Source: CAD feature listing. Evaluate the final solid. Frame: model axes, mm. A direction names the side the tool comes from. Coordinates: 2 decimals unless noted, no trailing zeros. Order: outer loops, then holes, each group sorted by start corner. A loop starts at its lowest first (then second) coordinate and runs counter-clockwise, first axis right, second up. Notation, with made-up numbers: (1.25, 27) -> (13.25, 27) arc R3 ccw to (13.25, 32) -> close; hole circle Ø3 at (21.5, 0). An arc over 180 degrees is marked (long way). Write item = value, one per line. Start each with the question number.
Item 1: Ray query, line 1 along X through (y, z) = (-7.25, -259); line 2 along X through (y, z) = (-26.5, 47.5). Return the intervals inside material, ascending. Write a range as [from, to].
Item 2: Section query B-B (z = -304). Output: boundary loops of the cut face in (x, y), then the cut area to 3 significant figures.
Item 3: Set-up query: faces 1 (the flat face through (30, -15, -228)), 2 (the flat face through (15, -15, -450)). Return all of +Z, -Z, +X, -X, +Y, -Y with unobstructed straight access to the full face (end or side cutting, diameter ignored); none if empty.
Item 4: Contact query for flat-ended pins moving along their axis: pin 1 (4 mm diameter, centred on x = 67.5, z = 369.5, fed in from +Y); pin 2 (10 mm diameter, centred on y = -10, z = 57, fed in from +X); pin 3 (9 mm diameter, centred on y = -5, z = -35.5, fed in from +X). Output: stop coordinate, or through.
Item 5: Section query A-A (y = -14.75). Output: boundary loops of the cut face in (x, z).
Item 6: Section query C-C (z = 126). Output: boundary loops of the cut face in (x, y), then the cut area to 3 significant figures.
```python
from build123d import *

# Parameters (mm, degrees)
F1_DEPTH = 30
F3_DEPTH = 8
F4_W     = 10
F4_H     = 30
F5_DEPTH = 8
F6_W     = 10
F6_H     = 30
F7_DEPTH = 8


with BuildPart() as f1:
    # F0 (on Front) → F1 (new body)
    with BuildSketch(Plane.XZ):
        Polygon((70.294598, 500), (0, 0), (0, -450), (30, -450), (30, 0), (100, 495.806066), align=None)
    extrude(amount=F1_DEPTH)

    # F2 (on face) → F3 (cut)
    with BuildSketch(Plane(origin=(0, 0, 0), x_dir=(-1, 0, 0), z_dir=(0, 1, 0))):
        Polygon((-73.234991, 449.086059), (-83.137606, 447.693859), (-80.353204, 427.888629), (-70.45059, 429.28083), align=None)
        Polygon((-63.489587, 379.767757), (-73.392201, 378.375556), (-70.6078, 358.570327), (-60.705185, 359.962527), align=None)
    extrude(amount=-F3_DEPTH, mode=Mode.SUBTRACT)

    # F4 (on face) → F5 (cut)
    with BuildSketch(Plane(origin=(0, 0, 0), x_dir=(-1, 0, 0), z_dir=(0, 1, 0))):
        with Locations((-15, -35)):
            Rectangle(F4_W, F4_H)
    extrude(amount=-F5_DEPTH, mode=Mode.SUBTRACT)

    # F6 (on face) → F7 (cut)
    with BuildSketch(Plane(origin=(0, 0, 0), x_dir=(0, -1, 0), z_dir=(-1, 0, 0))):
        with Locations((15, -35)):
            Rectangle(F6_W, F6_H)
    extrude(amount=-F7_DEPTH, mode=Mode.SUBTRACT)


solid = f1.part
```
Computed:
q1.line_1 = [0, 30]
q1.line_2 = [6.68, 36.71]
q2.outline = (0, -30) -> (30, -30) -> (30, 0) -> (0, 0) -> close
q2.area = 900 mm^2
q3.face_1 = -Z, +X, +Y, -Y
q3.face_2 = -Z, +X, -X, +Y, -Y
q4.pin_1 = -8
q4.pin_2 = 38.75
q4.pin_3 = 30
q5.outline = (0, -450) -> (30, -450) -> (30, 0) -> (100, 495.81) -> (70.29, 500) -> (0, 0) -> (0, -20) -> (8, -20) -> (8, -50) -> (0, -50) -> close
q6.outline = (17.71, -30) -> (47.79, -30) -> (47.79, 0) -> (17.71, 0) -> close
q6.area = 902 mm^2
